Autodesk Inventor part; units mm, degrees
ref_plane "YZ Plane" through (0, 0, 0) normal (1, 0, 0) x (0, 1, 0)
ref_plane "XZ Plane" through (0, 0, 0) normal (0, 1, 0) x (-1, 0, 0)
ref_plane "XY Plane" through (0, 0, 0) normal (0, 0, 1) x (1, 0, 0)
sketch "Sketch1" plane through (0, 0, 0) normal (0, 1, 0) x (-1, 0, 0)
  circle A0 centre (0, 0) radius 100.151
  line L0 (0, 0) -> (50.0755, -86.7333)
  line L1 (0, 0) -> (100.151, 0) construction
  line L2 (0, 0) -> (50.0755, 86.7333)
  line L3 (0, 0) -> (100.151, 0) construction
  line L4 (0, 0) -> (-100.151, 0)
  line L5 (50.0755, -86.7333) -> (100.0755, -86.7333) construction
  line L6 (50.0755, -86.7333) -> (24.5339, -97.0995)
  line L7 (50.0755, -86.7333) -> (100.0755, -86.7333) construction
  line L8 (71.8237, -69.7967) -> (50.0755, -86.7333)
  circle A1 centre (0, 0) radius 102.651
  line L9 (0, 0) -> (71.8237, -69.7967)
  line L10 (71.8237, -69.7967) -> (73.6166, -71.539)
  line L11 (0, 0) -> (24.5339, -97.0995)
  line L12 (24.5339, -97.0995) -> (25.1463, -99.5233)
  dimension "d0" = 200.302
  dimension "d1" = 60
  dimension "d2" = 60
  dimension "d8" = 205.302
extrude "Extrusion1" add sketch "Sketch1" along normal blind 40 contours L10 A1 L12 A0 picked at (67.2642, -76.2102)
sketch "Sketch2" plane through (0, 0, 0) normal (0, -1, 0) x (1, 0, 0)
  line L0 (-24.5339, -97.0995) -> (-25.1463, -99.5233)
  line L1 (-24.8401, -98.3114) -> (-21.9315, -99.0463)
  circle A0 centre (-21.9315, -99.0463) radius 1.5
  line L2 (-73.6166, -71.539) -> (-71.8237, -69.7967)
  line L3 (-72.7201, -70.6679) -> (-74.8716, -72.7586)
  line L4 (-74.8716, -72.7586) -> (-72.7201, -70.6679)
  line L5 (-72.7201, -70.6679) -> (-74.8109, -68.5164)
  circle A1 centre (-74.8109, -68.5164) radius 1.5
  circle A2 centre (-74.8109, -68.5164) radius 3
  arc A3 (-73.6166, -71.539) -> (-25.1463, -99.5233) centre (0, 0) ccw
  line L6 (-73.6166, -71.539) -> (-74.8109, -71.5164)
  arc A4 (-71.8237, -69.7967) -> (-24.5339, -97.0995) centre (0, 0) ccw
  line L7 (-71.8109, -68.5164) -> (-71.8237, -69.7967)
  circle A5 centre (-21.9315, -99.0463) radius 3
  line L8 (-21.9315, -99.0463) -> (-24.5296, -100.5463)
  line L9 (-21.9315, -99.0463) -> (-18.9315, -99.0463) construction
  line L10 (-24.5296, -100.5463) -> (-25.1463, -99.5233)
  arc A6 (-22.1585, -98.9889) -> (-21.9315, -99.0463) centre (-21.9315, -98.5684) ccw
  line L11 (-21.9315, -99.0463) -> (-22.9003, -97.4384)
  line L12 (-21.9315, -99.0463) -> (-20.0543, -99.0463) construction
  line L13 (-22.9003, -97.4384) -> (-23.4798, -96.4767)
  line L14 (-23.4798, -96.4767) -> (-24.5339, -97.0995)
  point P0 (0, 0)
  dimension "d12" = 3
  dimension "d13" = 3
  dimension "d14" = 3
  dimension "d15" = 210
  dimension "d16" = 121.07
extrude "Extrusion2" add sketch "Sketch2" against normal blind 3 contours L14 A5 L0 | L7 L2 A2 | A5 L10 L0 | A5 L13 L11 A0 L1 | L1 A0 L8 A5 | A5 L8 A0 L11 L13 | A0 L11 L1 | L1 A6 L8 A0 | L2 L6 A2 | A2 | L1 A6 | A0 L8 L11
sketch "Sketch3" plane through (0, 3, 0) normal (0, 1, 0) x (1, 0, 0)
  arc A0 (-23.4798, 96.4767) -> (-24.5296, 100.5463) centre (-21.9315, 99.0463) ccw
  circle A1 centre (-21.9315, 99.0463) radius 1.5
  point P0 (0, 0)
  dimension "d19" = 3
extrude "Extrusion3" cut sketch "Sketch3" against normal blind 3
properties part number "Wheel Guard"
Verification items for the finished model (mm, model axes). A direction names the side the tool comes from. Give positions to 0.01 mm unless a question says otherwise; leave off trailing zeros. Write each loop counter-clockwise with the first axis right and the second up, starting at its lowest first coordinate (ties: lowest second). Pieces come first, ordered by that corner, then holes.
(1) Gauge pin test, flat ends, axial feed: pin 1 (12 mm diameter, centred on x = -72, y = 31.5, fed in from +Z); pin 2 (1 mm diameter, centred on x = -51.5, y = 4.5, fed in from -Z); pin 3 (2 mm diameter, centred on y = 35, z = -87, fed in from +X). Record the tip position at first contact, or that the pin passes through.
(2) Mould release check, pull along Z, two halves, no side actions. Record for faces 4 (the face through (-21.125, 1.521, -100.311)), 5 (the face through (-19.053, 1.479, -99.891)), 6 (the face through (-76.31, 1.48, -68.45)), 7 (the face through (-74, 3, -67)): +Z half, -Z half, draft (parallel to the pull), parting line (faces both ways), or undercut.
(3) Cross-section at C-C (z = -73). Enter the section's corners in (x, y), plus the area to 3 significant figures.
(4) Cross-section at A-A (x = -22.5). Enter the section's corners in (y, z), plus the area to 3 significant figures.
(5) Access from +Z, -Z, +X, -X, +Y, -Y to the whole of each face (thin tool, end or side, straight path). Record for faces 1 (the face through (-24.836, 21.241, -98.294)), 2 (the face through (-72.71, 21.24, -70.66)), 3 (the face through (-49, 40, -88)).
(6) Cross-section at B-B (y = 7). Enter the section's corners in (x, z), plus the area to 3 significant figures.
(7) Material ranges on line 1 (Z direction, x = -46, y = 27); line 2 (Z direction, x = -41.5, y = 24); line 3 (X direction, y = 6, z = -84.5), recorded low to high.
(8) Cross-section at D-D (x = -72.5). Enter the section's corners in (y, z).
Worked out:
1. pin 1: stops at z = -69.8
1. pin 2: stops at z = -89.09
1. pin 3: stops at x = -47.81
2. face 4: undercut
2. face 5: parting line
2. face 6: undercut
2. face 7: draft
3. outline: (-72.17, 0) - (-68.57, 0) - (-68.57, 40) - (-72.17, 40) - close
3. area: 144 mm2
4. outline: (0, -101.99) - (3, -101.99) - (3, -100.43) - (0, -100.43) - close; (0, -97.66) - (3, -97.66) - (3, -96.1) - (0, -96.1) - close
4. area: 9.35 mm2
5. face 1: -Z, +X, +Y
5. face 2: +Z, -X, +Y
5. face 3: +Z, -Z, +X, -X, +Y
6. outline: (-73.62, -71.54) arc R102.65 ccw to (-25.15, -99.52) - (-24.53, -97.1) arc R100.15 cw to (-71.82, -69.8) - close
6. area: 140 mm2
7. line 1: z = -91.77 to -88.96
7. line 2: z = -93.89 to -91.15
7. line 3: x = -58.28 to -53.76
8. outline: (0, -72.67) - (40, -72.67) - (40, -70.45) - (3, -70.45) - (3, -66.6) - (0, -66.6) - close
